```python
from build123d import *

# Parameters (mm, degrees)
F0_W     = 10
F0_H     = 35.0110880776
F0_W_2   = 90
F0_R     = 5
F1_DEPTH = 2
F2_SIZE  = 1


with BuildPart() as f1:
    # F0 (on Front) → F1 (new body)
    with BuildSketch(Plane.XZ):
        with Locations((-50, 0)):
            Rectangle(F0_W, F0_H)
        Rectangle(F0_W_2, F0_H)
        with Locations((-35, 0)):
            Circle(F0_R, mode=Mode.SUBTRACT)
        with BuildLine():
            ThreePointArc((-26.5, 0), (-22.5, 4), (-18.5, 0))
            ThreePointArc((-18.5, 0), (-22.5, -4), (-26.5, 0))
        make_face(mode=Mode.SUBTRACT)
        with BuildLine():
            ThreePointArc((26.5, 0), (22.5, -4), (18.5, 0))
            ThreePointArc((18.5, 0), (22.5, 4), (26.5, 0))
        make_face(mode=Mode.SUBTRACT)
        with BuildLine():
            ThreePointArc((40, 0), (35, -5), (30, 0))
            ThreePointArc((30, 0), (35, 5), (40, 0))
        make_face(mode=Mode.SUBTRACT)
        with Locations((50, 0)):
            Rectangle(F0_W, F0_H)
    extrude(amount=-F1_DEPTH)

    # F2
    f2_edges = [f1.edges().sort_by_distance(p)[0] for p in [
        (55, 1, 17.505544),
        (55, 1, -17.505544),
        (-55, 1, -17.505544),
        (-55, 1, 17.505544),
    ]]
    chamfer(f2_edges, length=F2_SIZE)


solid = f1.part
```
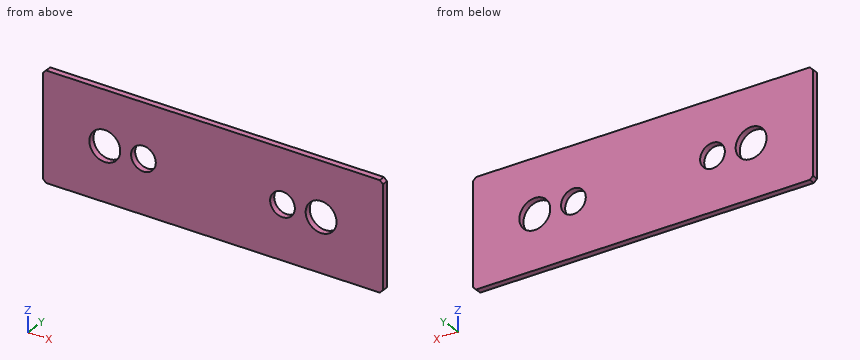
Verification items for the finished model (mm, model axes). Round coordinates to 2 decimals unless told otherwise and drop trailing zeros. Loops run counter-clockwise (first coordinate to the right, second up) from the corner with the lowest first, then second, coordinate; pieces in that order, holes last. Notation, with made-up numbers: (75, 43.25) -> (86, 43.25) arc R21 ccw to (86, 69.25) -> close; hole circle Ø6 at (65, -31.5). An arc over 180 degrees is marked (long way). Answer as a JSON object with one key per item and string values.
Q1. Scan lines: line 1 (X direction, y = 0.85, z = -0.5); line 2 (X direction, y = 1.6, z = 2); line 3 (Z direction, x = 22.5, y = 1). Record each from-to range of solid material in increasing order. Write a range as from..to.
Data:
{"line 1": "x = -55..-39.97, -30.03..-26.47, -18.53..18.53, 26.47..30.03, 39.97..55", "line 2": "x = -55..-39.58, -30.42..-25.96, -19.04..19.04, 25.96..30.42, 39.58..55", "line 3": "z = -17.51..-4, 4..17.51"}
Q2. Section check B-B (y = 0.95). Record the boundary of the cut face in (x, z).
Data:
{"outline": "(-55, -16.51) -> (-54, -17.51) -> (54, -17.51) -> (55, -16.51) -> (55, 16.51) -> (54, 17.51) -> (-54, 17.51) -> (-55, 16.51) -> close; hole circle Ø10 at (-35, 0); hole circle Ø8 at (-22.5, 0); hole circle Ø8 at (22.5, 0); hole circle Ø10 at (35, 0)"}
Q3. Section check A-A (x = -35). Record the boundary of the cut face in (y, z).
Data:
{"outline": "(0, -17.51) -> (2, -17.51) -> (2, -5) -> (0, -5) -> close; (0, 5) -> (2, 5) -> (2, 17.51) -> (0, 17.51) -> close"}
Q4. Section check C-C (x = -22.5). Record the boundary of the cut face in (y, z), then the cut area to 3 significant figures.
Data:
{"outline": "(0, -17.51) -> (2, -17.51) -> (2, -4) -> (0, -4) -> close; (0, 4) -> (2, 4) -> (2, 17.51) -> (0, 17.51) -> close", "area": "54.0 mm2"}
